Geometry check sheet. Reference: the model listing, model coordinates, mm. Face numbers are marked on the shaded views. Coordinates: 2 decimals unless noted, no trailing zeros. Write each loop counter-clockwise with the first axis right and the second up, starting at its lowest first coordinate (ties: lowest second). Pieces come first, ordered by that corner, then holes. Notation, with made-up numbers: (21, -22.5) -> (72, -22.5) arc R22 ccw to (72, -15.5) -> close; hole circle Ø8 at (42.5, 86.5). An arc over 180 degrees is marked (long way). Use a Markdown table: item, result.
```python
from build123d import *

# Parameters (mm, degrees)
F0_R     = 10.55
F0_R_2   = 10.05
F1_DEPTH = 3
F4_DEPTH = 2.5
F2_W     = 1
F2_H     = 0.45
F5_DEPTH = 2.5


with BuildPart() as f1:
    # F0 (on Top) → F1 (new body)
    with BuildSketch(Plane.XY):
        Circle(F0_R)
        Circle(F0_R_2, mode=Mode.SUBTRACT)
    extrude(amount=F1_DEPTH)

    # F3 (on face) → F4 (join)
    with BuildSketch(Plane(origin=(0, 0, 0), x_dir=(1, 0, 0), z_dir=(0, 0, -1))):
        Polygon((0, 10.05), (0.5, 10.05), (0.5, 10.5), (-0.5, 10.5), (-0.5, 10.05), align=None)
    extrude(amount=F4_DEPTH)

    # F2 (on Top) → F5 (join)
    with BuildSketch(Plane.XY):
        with Locations((0, 10.275)):
            Rectangle(F2_W, F2_H)
    extrude(amount=-F5_DEPTH)


solid = f1.part
```
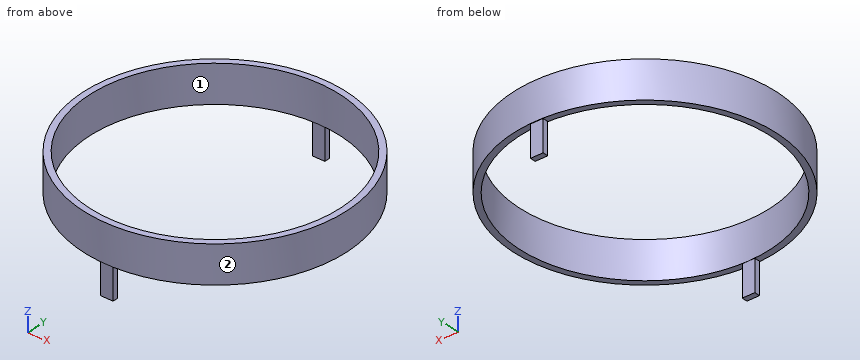
Item 1: Section check A-A on y = 0. Record the boundary of the cut face in (x, z), then the cut area to 3 significant figures.
Answer block:
| item | result |
|---|---|
| outline | (-10.55, 0) -> (-10.05, 0) -> (-10.05, 3) -> (-10.55, 3) -> close; (10.05, 0) -> (10.55, 0) -> (10.55, 3) -> (10.05, 3) -> close |
| area | 3.00 mm^2 |
Item 2: Thickness scan on L1, parallel to Y at x = 0, z = 1.7; L2, parallel to X at y = 9.25, z = 0.55; L3, parallel to X at y = -3.5, z = 1. Record the ranges inside material, lowest first. Write a range as [from, to].
Answer block:
| item | result |
|---|---|
| L1 | y = [-10.55, -10.05], [10.05, 10.55] |
| L2 | x = [-5.07, -3.93], [3.93, 5.07] |
| L3 | x = [-9.95, -9.42], [9.42, 9.95] |
Item 3: Section check C-C on z = 2.25. Record the boundary of the cut face in (x, y).
Answer block:
| item | result |
|---|---|
| outline | circle Ø21.1 at (0, 0); hole circle Ø20.1 at (0, 0) |
Item 4: Depth check by flat-ended pin: P1, Ø1, axis at x = -6, z = 1.5, coming from the -Y side; P2, Ø1.1, axis at x = 0, z = -1, coming from the +Y side; P3, Ø10, axis at x = 7.5, y = 1.5, coming from the -Z side; P4, Ø8, axis at x = 1, y = -7, coming from the +Z side. Enter the tip coordinate at first touch or a pass-through.
Answer block:
| item | result |
|---|---|
| P1 | stops at y = -9 |
| P2 | stops at y = 10.5 |
| P3 | stops at z = 0 |
| P4 | stops at z = 3 |
Item 5: Section check B-B on z = -0.45. Record the boundary of the cut face in (x, y).
Answer block:
| item | result |
|---|---|
| outline | (-0.5, -10.5) -> (0.5, -10.5) -> (0.5, -10.05) -> (-0.5, -10.05) -> close; (-0.5, 10.05) -> (0.5, 10.05) -> (0.5, 10.5) -> (-0.5, 10.5) -> close |
Item 6: Mould release check, pull along Y, two halves, no side actions. Record for the marked faces 1 and 2: +Y half, -Y half, draft (parallel to the pull), parting line (faces both ways), or undercut.
Answer block:
| item | result |
|---|---|
| face 1 | undercut |
| face 2 | parting line |
